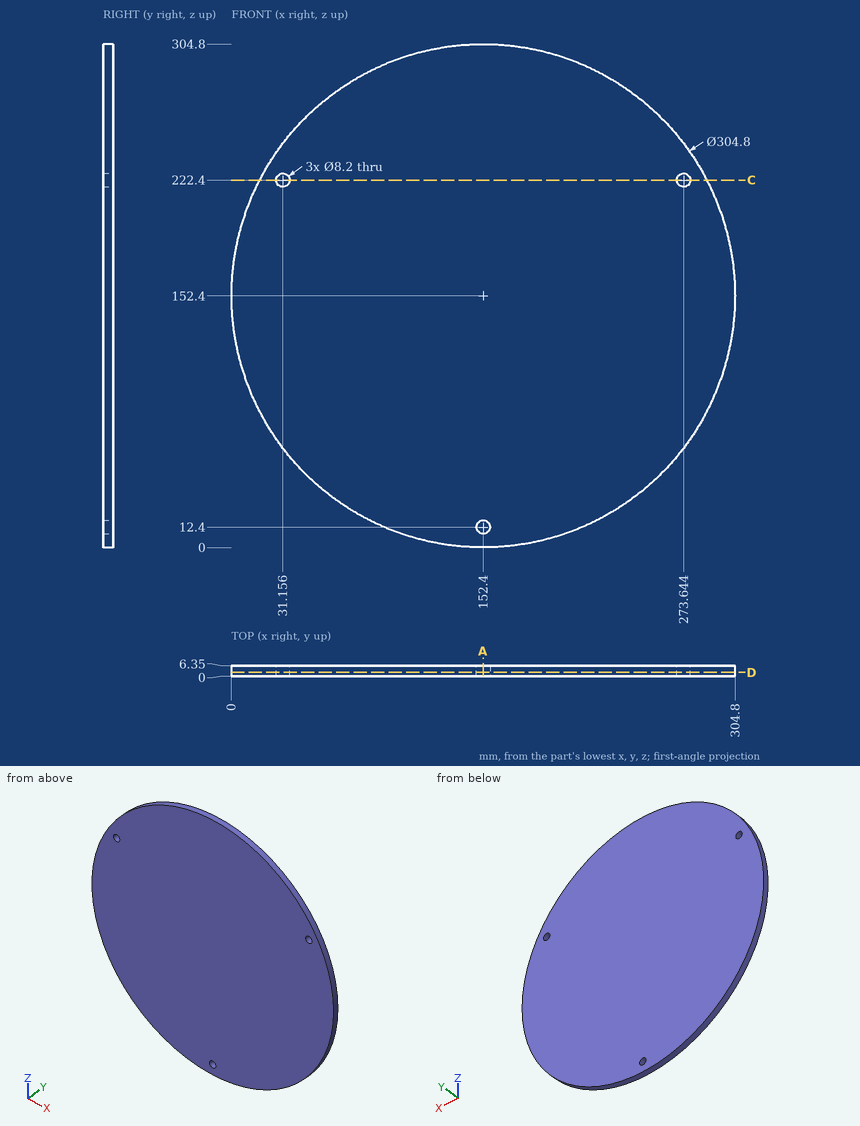
Here's the drawing with two shaded views (mm, measured from the low corner). I have some questions. Give positions to 0.01 mm unless a question says otherwise; leave off trailing zeros. Loops run counter-clockwise (first coordinate to the right, second up) from the corner with the lowest first, then second, coordinate; pieces in that order, holes last. Notation, with made-up numbers: M 59,62.5 L 70,62.5 A21 cw 70,83.5 Z; hole C 52,3.5 d11. An arc over 180 degrees is marked long. Answer in a Markdown table with one row per item.
1. If I drill on line 1 along Z through (x, y) = (152.4, 1.5); line 2 along Z through (x, y) = (33, 1.75) (1 decimal); line 3 along X through (y, z) = (3, 14) (1 decimal), over which ranges is the centre line in solid material (lowest first)?
Taken from the geometry:
| item | result |
|---|---|
| line 1 | z = 0 to 8.3, 16.5 to 304.8 |
| line 2 | z = 57.7 to 218.7, 226.1 to 247.1 |
| line 3 | x = 88.6 to 148.6, 156.2 to 216.2 |
2. Suppose I cut it at C-C on z = 222.4. Write out the boundary of the cut face in (x, y).
Taken from the geometry:
| item | result |
|---|---|
| outline | M 17.03,0 L 27.06,0 L 27.06,6.35 L 17.03,6.35 Z; M 35.26,0 L 269.54,0 L 269.54,6.35 L 35.26,6.35 Z; M 277.74,0 L 287.77,0 L 287.77,6.35 L 277.74,6.35 Z |
3. Suppose I cut it at A-A on x = 152.4. Write out the boundary of the cut face in (y, z), plus the area to 3 significant figures.
Taken from the geometry:
| item | result |
|---|---|
| outline | M 0,0 L 6.35,0 L 6.35,8.3 L 0,8.3 Z; M 0,16.5 L 6.35,16.5 L 6.35,304.8 L 0,304.8 Z |
| area | 1,880 mm² |
4. Suppose I cut it at D-D on y = 2.25. Write out the boundary of the cut face in (x, z), plus the area to 3 significant figures.
Taken from the geometry:
| item | result |
|---|---|
| outline | C 152.4,152.4 d304.8; hole C 31.16,222.4 d8.2; hole C 152.4,12.4 d8.2; hole C 273.64,222.4 d8.2 |
| area | 72,800 mm² |
5. For pin 1 Ø4 at (x, z) = (75, 202.5) entering from -Y; pin 2 Ø2 at (y, z) = (3, 93.5) entering from +X; pin 3 Ø1.5 at (y, z) = (1, 114) entering from -X, each with a flat end and sliding along its axis, tell me the tip position at first contact or that it passes through.
Taken from the geometry:
| item | result |
|---|---|
| pin 1 | stops at y = 0 |
| pin 2 | stops at x = 293.37 |
| pin 3 | stops at x = 4.72 |
